CAD build for the part. Positions are in the model's coordinates, mm. Round coordinates to 2 decimals unless told otherwise and drop trailing zeros. Write each loop counter-clockwise with the first axis right and the second up, starting at its lowest first coordinate (ties: lowest second). Pieces come first, ordered by that corner, then holes. Notation, with made-up numbers: (24.5, 27.5) - (37.5, 27.5) arc R29 cw to (37.5, 64.5) - close; hole circle Ø1 at (47.5, -20.75). An arc over 180 degrees is marked (long way). Answer in a Markdown table with one row per item.
Autodesk Inventor part; units mm, degrees
ref_plane "YZ Plane" through (0, 0, 0) normal (1, 0, 0) x (0, 1, 0)
ref_plane "XZ Plane" through (0, 0, 0) normal (0, 1, 0) x (-1, 0, 0)
ref_plane "XY Plane" through (0, 0, 0) normal (0, 0, 1) x (1, 0, 0)
sketch "スケッチ1" plane through (0, 0, 0) normal (0, 1, 0) x (-1, 0, 0)
  circle A0 centre (0, 0) radius 12.5
  line L0 (-15, -45) -> (-15, 45)
  line L1 (-15, 45) -> (15, 45)
  line L2 (15, 45) -> (15, -45)
  line L3 (15, -45) -> (-15, -45)
  line L4 (-15, -45) -> (15, 45) construction
  line L5 (-15, 45) -> (15, -45) construction
  circle A1 centre (0, -8.5) radius 1.5
  circle A2 centre (0, 8.5) radius 1.5
  dimension "d0" = 25
  dimension "d1" = 90
  dimension "d2" = 30
  dimension "d10" = 3
  dimension "d11" = 3
extrude "押し出し3" add sketch "スケッチ1" along normal blind 3 contours A0 | L0 L1 L2 L3
sketch "スケッチ3" plane through (0, 3, 0) normal (0, 1, 0) x (1, 0, 0)
  circle A0 centre (0, 0) radius 3.75
  dimension "d14" = 7.5
extrude "押し出し4" cut sketch "スケッチ3" against normal blind 3
sketch "スケッチ4" plane through (0, 3, 0) normal (0, 1, 0) x (1, 0, 0)
  line L0 (0, 0) -> (0, 30)
  line L1 (0, 30) -> (0, -30)
  line L2 (0, -30) -> (-9, -30)
  line L3 (-15, 45) -> (-15, -45)
  circle A0 centre (-9, -30) radius 2.5
  line L4 (0, -30) -> (9, -30)
  line L5 (9, -30) -> (-9, 30)
  line L6 (-9, -30) -> (9, 30)
  circle A1 centre (9, -30) radius 2.5
  circle A2 centre (-9, 30) radius 2.5
  circle A3 centre (9, 30) radius 2.5
  dimension "d17" = 30
  dimension "d18" = 60
  dimension "d19" = 9
  dimension "d20" = 5
  dimension "d21" = 9
  dimension "d23" = 5
  dimension "d24" = 5
  dimension "d25" = 5
extrude "押し出し5" cut sketch "スケッチ4" against normal blind 3 contours A2 | A3 | A1 L4 L5 | L5 L4 A1 | L6 L2 A0 | A0 L2 L6
properties part number "板 中心Φ7" material "アルミニウム 6061"
Q1. Saw through at C-C on x = 0. List the corners of the cut face in (y, z), then the cut area to 4 significant figures.
Computed:
| item | result |
|---|---|
| outline | (0, -45) - (3, -45) - (3, -10) - (0, -10) - close; (0, -7) - (3, -7) - (3, -3.75) - (0, -3.75) - close; (0, 3.75) - (3, 3.75) - (3, 7) - (0, 7) - close; (0, 10) - (3, 10) - (3, 45) - (0, 45) - close |
| area | 229.5 mm2 |
Q2. Saw through at D-D on y = 0.6. List the corners of the cut face in (x, z), then the cut area to 3 significant figures.
Computed:
| item | result |
|---|---|
| outline | (-15, -45) - (15, -45) - (15, 45) - (-15, 45) - close; hole circle Ø5 at (-9, -30); hole circle Ø5 at (-9, 30); hole circle Ø7.5 at (0, 0); hole circle Ø3 at (0, -8.5); hole circle Ø3 at (0, 8.5); hole circle Ø5 at (9, -30); hole circle Ø5 at (9, 30) |
| area | 2,560 mm2 |
Q3. Flat gauge pin, fed straight in: pin 1 (4.5 mm diameter, centred on x = 0, z = 0, fed in from +Y). Where does the tip first touch, or does it go through?
Computed:
| item | result |
|---|---|
| pin 1 | passes through |
Q4. Saw through at B-B on z = 30. List the corners of the cut face in (x, y).
Computed:
| item | result |
|---|---|
| outline | (-15, 0) - (-11.5, 0) - (-11.5, 3) - (-15, 3) - close; (-6.5, 0) - (6.5, 0) - (6.5, 3) - (-6.5, 3) - close; (11.5, 0) - (15, 0) - (15, 3) - (11.5, 3) - close |
Q5. Drill centre lines: line 1 (X direction, y = 1.2, z = -30); line 2 (Z direction, x = -9, y = 2.05); line 3 (Z direction, x = 0, y = 1.7). Where is each one in solid material? Low to high.
Computed:
| item | result |
|---|---|
| line 1 | x = -15 to -11.5, -6.5 to 6.5, 11.5 to 15 |
| line 2 | z = -45 to -32.5, -27.5 to 27.5, 32.5 to 45 |
| line 3 | z = -45 to -10, -7 to -3.75, 3.75 to 7, 10 to 45 |
Q6. Saw through at A-A on x = 10.5. List the corners of the cut face in (y, z).
Computed:
| item | result |
|---|---|
| outline | (0, -45) - (3, -45) - (3, -32) - (0, -32) - close; (0, -28) - (3, -28) - (3, 28) - (0, 28) - close; (0, 32) - (3, 32) - (3, 45) - (0, 45) - close |
Q7. Pull direction Z, two halves, no side cores. Call faces 1 (the flat face through (-15, 1, 1)), 2 (the cylindrical face through (-7.66, 1.52, -32.11)), 3 (the flat face through (0, 1, 45)): released by +Z, released by -Z, zero draft, split by the parting line, or undercut.
Computed:
| item | result |
|---|---|
| face 1 | zero draft |
| face 2 | undercut |
| face 3 | released by +Z |
